Build history of the part. All positions in model axes, mm. Face numbers are marked on the shaded views. A direction names the side the tool comes from. Round coordinates to 2 decimals unless told otherwise and drop trailing zeros. Write each loop counter-clockwise with the first axis right and the second up, starting at its lowest first coordinate (ties: lowest second). Pieces come first, ordered by that corner, then holes. Notation, with made-up numbers: (72.5, 53.25) -> (79.5, 53.25) arc R27 cw to (79.5, 77.25) -> close; hole circle Ø6 at (10, 41.5). An arc over 180 degrees is marked (long way). Return JSON: item names as keys, results as strings.
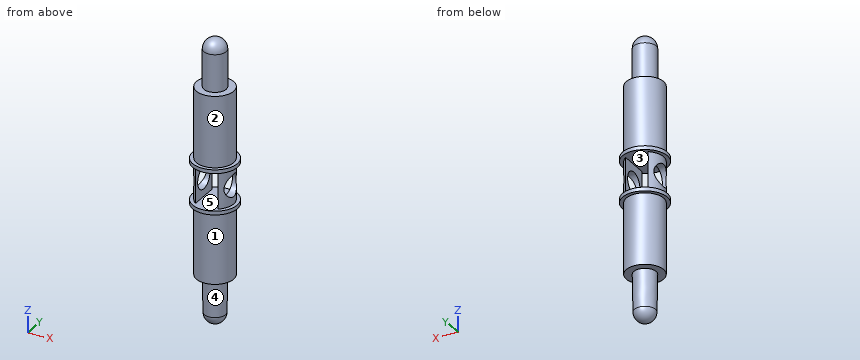
from build123d import *

# Parameters (mm, degrees)
SKETCH2_R               = 5
BOSS_EXTRUDE1_DEPTH     = 50
SKETCH3_R               = 3
BOSS_EXTRUDE2_DEPTH     = 10
BOSS_EXTRUDE2_TAPER     = 1
SKETCH5_R               = 3
BOSS_EXTRUDE3_DEPTH     = 10
SKETCH7_W               = 6
SKETCH7_H               = 10
CUT_EXTRUDE1_DEPTH      = 10
CUT_EXTRUDE1_DEPTH_BACK = 10
SKETCH8_R               = 3
CUT_EXTRUDE2_DEPTH      = 10
CUT_EXTRUDE2_DEPTH_BACK = 10
SKETCH10_R              = 6
BOSS_EXTRUDE4_DEPTH     = 1
SKETCH11_R              = 6
BOSS_EXTRUDE5_DEPTH     = 1


with BuildPart() as part:
    # Sketch2 → Boss-Extrude1 (new body)
    with BuildSketch(Plane.XY):
        Circle(SKETCH2_R)
    extrude(amount=BOSS_EXTRUDE1_DEPTH)

    # Sketch3 → Boss-Extrude2 (add)
    with BuildSketch(Plane(origin=(0, 0, 0), x_dir=(-1, 0, 0), z_dir=(0, 0, -1))):
        Circle(SKETCH3_R)
    extrude(amount=BOSS_EXTRUDE2_DEPTH, taper=BOSS_EXTRUDE2_TAPER)

    # Sketch5 → Boss-Extrude3 (add)
    with BuildSketch(Plane.XY.offset(50)):
        Circle(SKETCH5_R)
    extrude(amount=BOSS_EXTRUDE3_DEPTH)

    # Sketch7 → Cut-Extrude1 (cut, two sides)
    with BuildSketch(Plane(origin=(0, 0, 0), x_dir=(1, 0, 0), z_dir=(0, 1, 0))) as cut_extrude1_sk:
        with Locations((0, -25)):
            Rectangle(SKETCH7_W, SKETCH7_H)
    extrude(amount=CUT_EXTRUDE1_DEPTH, mode=Mode.SUBTRACT)
    extrude(cut_extrude1_sk.sketch, amount=-CUT_EXTRUDE1_DEPTH_BACK, mode=Mode.SUBTRACT)

    # Sketch8 → Cut-Extrude2 (cut, two sides)
    with BuildSketch(Plane(origin=(0, 0, 0), x_dir=(0, 0, -1), z_dir=(1, 0, 0))) as cut_extrude2_sk:
        with Locations((-25, 0)):
            Circle(SKETCH8_R)
    extrude(amount=CUT_EXTRUDE2_DEPTH, mode=Mode.SUBTRACT)
    extrude(cut_extrude2_sk.sketch, amount=-CUT_EXTRUDE2_DEPTH_BACK, mode=Mode.SUBTRACT)

    # Sketch6 → Revolve1 (revolve)
    with BuildSketch(Plane.XY.offset(60)):
        with BuildLine():
            Line((0, 3), (0, -3))
            ThreePointArc((0, -3), (-3, 0), (0, 3))
        make_face()
    revolve(axis=Axis((0, 3, 60), (0, -1, 0)))

    # Sketch4 → Revolve2 (revolve)
    with BuildSketch(Plane(origin=(0, 0, -10), x_dir=(-1, 0, 0), z_dir=(0, 0, -1))):
        with BuildLine():
            Line((0, 2.825449351), (0, -2.825449351))
            ThreePointArc((0, -2.825449351), (-2.825449351, 0), (0, 2.825449351))
        make_face()
    revolve(axis=Axis((0, 2.825449351, -10), (0, -1, 0)))

    # Sketch10 → Boss-Extrude4 (add)
    with BuildSketch(Plane.XY.offset(20)):
        Circle(SKETCH10_R)
    extrude(amount=-BOSS_EXTRUDE4_DEPTH)

    # Sketch11 → Boss-Extrude5 (add)
    with BuildSketch(Plane.XY.offset(30)):
        Circle(SKETCH11_R)
    extrude(amount=BOSS_EXTRUDE5_DEPTH)


solid = part.part
Q1. Saw through at B-B on z = 52. List the corners of the cut face in (x, y).
Verdict:
{"outline": "circle Ø6 at (0, 0)"}
Q2. Wall check: L1, parallel to Z at x = -3.25, y = 4.5; L2, parallel to Z at x = 3.5, y = 0; L3, parallel to X at y = 3, z = 18. Give the ranges that are in metal, low to high.
Verdict:
{"L1": "z = 19 to 20, 30 to 31", "L2": "z = 0 to 22, 28 to 50", "L3": "x = -4 to 4"}
Q3. Saw through at A-A on z = 25. List the corners of the cut face in (x, y), then the cut area to 3 significant figures.
Verdict:
{"outline": "(-4, -3) arc R5 ccw to (-3, -4) -> (-3, -3) -> close; (-4, 3) -> (-3, 3) -> (-3, 4) arc R5 ccw to start; (3, -4) arc R5 ccw to (4, -3) -> (3, -3) -> close; (3, 3) -> (4, 3) arc R5 ccw to (3, 4) -> close", "area": "2.19 mm²"}
Q4. 3-axis set-ups, long thin cutter, end or side, ignore diameter. For the marked faces 1 and 2: which of +Z, -Z, +X, -X, +Y, -Y reach the whole face in a straight line?
Verdict:
{"face 1": "-Z", "face 2": "+Z"}
Q5. Pin check, flat tips, straight feed: pin 1 Ø1.5 at (x, y) = (-3.5, 4.5) entering from +Z; pin 2 Ø2.5 at (y, z) = (1, 26) entering from +X; pin 3 Ø6.5 at (y, z) = (-1.5, 24.5) entering from -X; pin 4 Ø3.5 at (x, y) = (2.5, 1.5) entering from -Z. Stop position of each tip, or through.
Verdict:
{"pin 1": "stops at z = 50", "pin 2": "passes through", "pin 3": "stops at x = -5", "pin 4": "stops at z = -12.57"}
Q6. Two-plate mould, pull along X, no slides. Class the marked faces 3, 4 and 5: +X half, -X half, draft (parallel to the pull), parting line (faces both ways), or undercut.
Verdict:
{"face 3": "undercut", "face 4": "parting line", "face 5": "undercut"}
